The model under review builds one solid part; all positions refer to its coordinate system, in mm. A direction names the side the tool comes from. Coordinates: 2 decimals unless noted, no trailing zeros. Order: outer loops, then holes, each group sorted by start corner. A loop starts at its lowest first (then second) coordinate and runs counter-clockwise, first axis right, second up. Notation, with made-up numbers: M -25.5,-19 L 19.5,-19 A35 ccw 19.5,17 Z; hole C 15,70 d7. An arc over 180 degrees is marked long. One line per item, written item: value.
```python
from build123d import *

# Parameters (mm, degrees)
SKETCH1_W           = 221
SKETCH1_H           = 45
BOSS_EXTRUDE1_DEPTH = 5
SKETCH2_W           = 211
SKETCH2_H           = 25
CUT_EXTRUDE1_DEPTH  = 2.5
SKETCH3_R           = 8
CUT_EXTRUDE2_DEPTH  = 2.5
SKETCH6_W           = 221
SKETCH6_H           = 45
SKETCH6_W_2         = 216
SKETCH6_H_2         = 40
BOSS_EXTRUDE3_DEPTH = 30
SKETCH7_W           = 7
SKETCH7_H           = 7.5
BOSS_EXTRUDE4_DEPTH = 17.5
SKETCH9_R           = 1
CUT_EXTRUDE3_DEPTH  = 6


with BuildPart() as part:
    # Sketch1 → Boss-Extrude1 (new body)
    with BuildSketch(Plane(origin=(0, 0, 0), x_dir=(1, 0, 0), z_dir=(0, 1, 0))):
        Rectangle(SKETCH1_W, SKETCH1_H)
    extrude(amount=BOSS_EXTRUDE1_DEPTH)

    # Sketch2 → Cut-Extrude1 (cut)
    with BuildSketch(Plane(origin=(0, 5, 0), x_dir=(1, 0, 0), z_dir=(0, 1, 0))):
        Rectangle(SKETCH2_W, SKETCH2_H)
    extrude(amount=-CUT_EXTRUDE1_DEPTH, mode=Mode.SUBTRACT)

    # Sketch3 → Cut-Extrude2 (cut)
    with BuildSketch(Plane(origin=(0, 2.5, 0), x_dir=(1, 0, 0), z_dir=(0, 1, 0))):
        with Locations(Location((-53, 0, 0), (0, 0, 270))):
            Circle(SKETCH3_R)
        with Locations(Location((53, 0, 0), (0, 0, 270))):
            Circle(SKETCH3_R)
    extrude(amount=-CUT_EXTRUDE2_DEPTH, mode=Mode.SUBTRACT)

    # Sketch6 → Boss-Extrude3 (add)
    with BuildSketch(Plane(origin=(0, 5, 0), x_dir=(1, 0, 0), z_dir=(0, 1, 0))):
        Rectangle(SKETCH6_W, SKETCH6_H)
        Rectangle(SKETCH6_W_2, SKETCH6_H_2, mode=Mode.SUBTRACT)
    extrude(amount=BOSS_EXTRUDE3_DEPTH)

    # Sketch7 → Boss-Extrude4 (add)
    with BuildSketch(Plane(origin=(0, 5, 0), x_dir=(1, 0, 0), z_dir=(0, 1, 0))):
        with Locations((-89, 16.25)):
            Rectangle(SKETCH7_W, SKETCH7_H)
        with Locations((-89, -16.25)):
            Rectangle(SKETCH7_W, SKETCH7_H)
        with Locations((-16.5, 16.25)):
            Rectangle(SKETCH7_W, SKETCH7_H)
        with Locations((-16.5, -16.25)):
            Rectangle(SKETCH7_W, SKETCH7_H)
        with Locations((16.5, 16.25)):
            Rectangle(SKETCH7_W, SKETCH7_H)
        with Locations((16.5, -16.25)):
            Rectangle(SKETCH7_W, SKETCH7_H)
        with Locations((89, 16.25)):
            Rectangle(SKETCH7_W, SKETCH7_H)
        with Locations((89, -16.25)):
            Rectangle(SKETCH7_W, SKETCH7_H)
    extrude(amount=BOSS_EXTRUDE4_DEPTH)

    # Sketch9 → Cut-Extrude3 (cut)
    with BuildSketch(Plane(origin=(0, 22.5, 0), x_dir=(1, 0, 0), z_dir=(0, 1, 0))):
        with Locations(Location((-89, 16, 0), (0, 0, 270))):
            Circle(SKETCH9_R)
        with Locations(Location((-89, -16, 0), (0, 0, 270))):
            Circle(SKETCH9_R)
        with Locations(Location((-16.5, 16, 0), (0, 0, 270))):
            Circle(SKETCH9_R)
        with Locations(Location((-16.5, -16, 0), (0, 0, 270))):
            Circle(SKETCH9_R)
        with Locations(Location((16.5, 16, 0), (0, 0, 270))):
            Circle(SKETCH9_R)
        with Locations(Location((16.5, -16, 0), (0, 0, 270))):
            Circle(SKETCH9_R)
        with Locations(Location((89, 16, 0), (0, 0, 270))):
            Circle(SKETCH9_R)
        with Locations(Location((89, -16, 0), (0, 0, 270))):
            Circle(SKETCH9_R)
    extrude(amount=-CUT_EXTRUDE3_DEPTH, mode=Mode.SUBTRACT)


solid = part.part
```
(1) We need section D-D, the plane x = -48.5. State the section outline as (y, z) points, plus the area to 3 significant figures.
Geometry results:
outline: M 0,-22.5 L 35,-22.5 L 35,-20 L 5,-20 L 5,-12.5 L 2.5,-12.5 L 2.5,-6.61 L 0,-6.61 Z; M 0,6.61 L 2.5,6.61 L 2.5,12.5 L 5,12.5 L 5,20 L 35,20 L 35,22.5 L 0,22.5 Z
area: 279 mm2
(2) We need section C-C, the plane y = 28.5. State the section outline as (x, z) points, plus the area to 4 significant figures.
Geometry results:
outline: M -110.5,-22.5 L 110.5,-22.5 L 110.5,22.5 L -110.5,22.5 Z; hole M -108,-20 L 108,-20 L 108,20 L -108,20 Z
area: 1,305 mm2
(3) For L1, parallel to X at y = 21, z = -14; L2, parallel to X at y = 1.15, z = 0; L3, parallel to X at y = 7, z = 1.5, list the stretches that pass through material, from the lowest coordinate up.
Geometry results:
L1: x = -110.5 to -108, -92.5 to -85.5, -20 to -13, 13 to 20, 85.5 to 92.5, 108 to 110.5
L2: x = -110.5 to -61, -45 to 45, 61 to 110.5
L3: x = -110.5 to -108, 108 to 110.5
(4) We need section B-B, the plane z = 0. State the section outline as (x, y) points, plus the area to 4 significant figures.
Geometry results:
outline: M -110.5,0 L -61,0 L -61,2.5 L -105.5,2.5 L -105.5,5 L -108,5 L -108,35 L -110.5,35 Z; M -45,0 L 45,0 L 45,2.5 L -45,2.5 Z; M 61,0 L 110.5,0 L 110.5,35 L 108,35 L 108,5 L 105.5,5 L 105.5,2.5 L 61,2.5 Z
area: 647.5 mm2
(5) We need section A-A, the plane x = 53. State the section outline as (y, z) points.
Geometry results:
outline: M 0,-22.5 L 35,-22.5 L 35,-20 L 5,-20 L 5,-12.5 L 2.5,-12.5 L 2.5,-8 L 0,-8 Z; M 0,8 L 2.5,8 L 2.5,12.5 L 5,12.5 L 5,20 L 35,20 L 35,22.5 L 0,22.5 Z
(6) Mouldability with a two-part tool opening along Z and no side actions: class faces 3 (the flat face through (-2, 0, 0)), 4 (the flat face through (88, 22.5, 17)), 5 (the flat face through (-2, 17, -22.5)) as +Z half, -Z half, draft (parallel to the pull), parting line (faces both ways), or undercut.
Geometry results:
face 3: draft
face 4: undercut
face 5: -Z half
(7) Insertion check: pin 1 Ø0.6 at (x, z) = (-16.5, -16.5) entering from +Y; pin 2 Ø1.5 at (x, z) = (-70.5, -13) entering from -Y; pin 3 Ø4 at (x, z) = (82.5, 3.5) entering from +Y; pin 4 Ø2 at (x, z) = (-45.5, 14.5) entering from +Y. Each pin has a flat end and moves straight along its axis. Give the tip position at first contact, or say it passes through.
Geometry results:
pin 1: stops at y = 16.5
pin 2: stops at y = 0
pin 3: stops at y = 2.5
pin 4: stops at y = 5
(8) Tool access review of faces 1 (the flat face through (13, 14, -16)), 2 (the flat face through (-110.5, 17, 0)): name each direction out of +Z, -Z, +X, -X, +Y, -Y from which nothing blocks a thin tool from reaching the whole face with its end or side.
Geometry results:
face 1: +Y
face 2: +Z, -Z, -X, +Y, -Y
